Design review of the part built by this model. Coordinates are the model's own, in mm. A direction names the side the tool comes from. Give positions to 0.01 mm unless a question says otherwise; leave off trailing zeros. Loops run counter-clockwise (first coordinate to the right, second up) from the corner with the lowest first, then second, coordinate; pieces in that order, holes last.
from build123d import *

# Parameters (mm, degrees)
CROQUIS1_R              = 52.6
SALIENTE_EXTRUIR1_DEPTH = 75.4
CROQUIS3_R              = 10
CROQUIS2_R              = 52.6
CROQUIS4_R              = 10
SALIENTE_EXTRUIR2_DEPTH = 30
CROQUIS7_R              = 17.5
CORTAR_EXTRUIR2_DEPTH   = 24


# Read off the part's stored shape, not the designer's step: Vaciado2
with BuildPart() as part:
    # Croquis1 → Saliente-Extruir1 (new body)
    with BuildSketch(Plane(origin=(0, 0, 0), x_dir=(1, 0, 0), z_dir=(0, 1, 0))):
        with Locations(Location((0, 0, 0), (0, 0, 270))):
            Circle(CROQUIS1_R)
    extrude(amount=-SALIENTE_EXTRUIR1_DEPTH)

    # Croquis3 → Recubrir1 section 0
    with BuildSketch(Plane(origin=(0, -121.9, 0), x_dir=(1, 0, 0), z_dir=(0, 1, 0))):
        Circle(CROQUIS3_R)
    # Croquis2 → Recubrir1 section 1
    with BuildSketch(Plane.XZ.offset(75.4)):
        Circle(CROQUIS2_R)
    loft()

    # Croquis4 → Saliente-Extruir2 (add)
    with BuildSketch(Plane.XZ.offset(121.9)):
        with Locations(Location((0, 0, 0), (0, 0, 270))):
            Circle(CROQUIS4_R)
    extrude(amount=SALIENTE_EXTRUIR2_DEPTH)

    # Croquis7 → Cortar-Extruir2 (cut)
    with BuildSketch(Plane.XZ.offset(151.9)):
        Circle(CROQUIS7_R)
    extrude(amount=-CORTAR_EXTRUIR2_DEPTH, mode=Mode.SUBTRACT)

    # Vaciado2 outline → Vaciado2 (revolve, cut)
    with BuildSketch(Plane.XY):
        Polygon((0, -127.9), (6.825, -127.9), (6.825, -120.665510856), (49.425, -74.165510856), (49.425, 0), (0, 0), align=None)
    revolve(axis=Axis((0, 0, 0), (0, 1, 0)), mode=Mode.SUBTRACT)


solid = part.part
Q1. Draft analysis for pull direction X (two halves, no side actions). For faces 4 (the face through (-3.8, -113.8, 17)), 5 (the face through (47, 0, -16)), 6 (the face through (13.566, -112.59, -4.272)), state which applies: pulls with the +X half, pulls with the -X half, needs draft (parallel to the pull), parting line crosses it, or undercut.
Results:
face 4: parting line crosses it
face 5: needs draft
face 6: undercut
Q2. Insertion check: pin 1 (10 mm diameter, centred on y = -65.5, z = 29.5, fed in from +X); pin 2 (1.5 mm diameter, centred on x = 0.5, z = 34.5, fed in from -Y); pin 3 (15.5 mm diameter, centred on x = 0, z = 0, fed in from +Y); pin 4 (6 mm diameter, centred on x = 0.5, y = -15, fed in from +Z). Each pin has a flat end and moves straight along its axis. Give the tip position at first contact, or say it passes through.
Results:
pin 1: stops at x = 46.55
pin 2: stops at y = -95.97
pin 3: stops at y = -119.66
pin 4: stops at z = 52.6
Q3. Take a section at A-A (x = 0). Give the boundary of the cut face in (y, z) (3 decimals).
Results:
outline: (-127.9, -10) - (-121.9, -10) - (-75.4, -52.6) - (0, -52.6) - (0, -49.425) - (-74.166, -49.425) - (-120.666, -6.825) - (-127.9, -6.825) - close; (-127.9, 6.825) - (-120.666, 6.825) - (-74.166, 49.425) - (0, 49.425) - (0, 52.6) - (-75.4, 52.6) - (-121.9, 10) - (-127.9, 10) - close
Q4. Take a section at B-B (y = -55). Give the boundary of the cut face in (x, z) (3 decimals), plus the area to 3 significant figures.
Results:
outline: circle Ø105.2 at (0, 0); hole circle Ø98.85 at (0, 0)
area: 1,020 mm2
Q5. Tool access review of faces 1 (the face through (-10.71, -36.56, 48.25)), 2 (the face through (7, -127.9, -2)), 3 (the face through (-9.76, -124.86, 2.17)): name each direction out of +Z, -Z, +X, -X, +Y, -Y from which nothing blocks a thin tool from reaching the whole face with its end or side.
Results:
face 1: +Y
face 2: +Z, -Z, +X, -X, -Y
face 3: -Y
Q6. Wall thickness on line 1 (X direction, y = -16.5, z = 0) (3 decimals); line 2 (X direction, y = -123, z = 0) (3 decimals): over which ranges is each line inside the solid? List them lowest first.
Results:
line 1: x = -52.6 to -49.425, 49.425 to 52.6
line 2: x = -10 to -6.825, 6.825 to 10
